from build123d import *

# Parameters (mm, degrees)
SKETCH1_W            = 70
SKETCH1_H            = 40
BOSS_EXTRUDE1_DEPTH  = 5
SKETCH2_W            = 90
SKETCH2_H            = 40
BOSS_EXTRUDE2_DEPTH  = 3
M3_CLEARANCE_HOLE1_D = 3.6
M3_CLEARANCE_HOLE2_D = 3.4
SKETCH9_R            = 14
CUT_EXTRUDE1_DEPTH   = 50.889878733
SKETCH10_W           = 40
SKETCH10_H           = 5
CUT_EXTRUDE2_DEPTH   = 0.5


with BuildPart() as part:
    # Sketch1 → Boss-Extrude1 (new body)
    with BuildSketch(Plane(origin=(0, 0, 0), x_dir=(1, 0, 0), z_dir=(0, 1, 0))):
        Rectangle(SKETCH1_W, SKETCH1_H)
    extrude(amount=BOSS_EXTRUDE1_DEPTH)

    # Sketch2 → Boss-Extrude2 (add)
    with BuildSketch(Plane.XZ):
        Rectangle(SKETCH2_W, SKETCH2_H)
    extrude(amount=BOSS_EXTRUDE2_DEPTH)

    # M3 Clearance Hole1 (through all)
    with Locations(Plane(origin=(0, 0, 0), x_dir=(1, 0, 0), z_dir=(0, 1, 0))):
        with Locations((-40, 15), (-40, -15), (40, 15), (40, -15)):
            Hole(M3_CLEARANCE_HOLE1_D / 2)

    # M3 Clearance Hole2 (through all)
    with Locations(Plane(origin=(0, 5, 0), x_dir=(1, 0, 0), z_dir=(0, 1, 0))):
        with Locations((0, 0), (15.25, 15.25), (-15.25, -15.25), (-15.25, 15.25), (15.25, -15.25)):
            Hole(M3_CLEARANCE_HOLE2_D / 2)

    # Sketch9 → Cut-Extrude1 (cut, through all)
    with BuildSketch(Plane(origin=(0, 5, 0), x_dir=(1, 0, 0), z_dir=(0, 1, 0))):
        with Locations(Location((0, 0, 0), (0, 0, 270))):
            Circle(SKETCH9_R)
    extrude(amount=-CUT_EXTRUDE1_DEPTH, mode=Mode.SUBTRACT)

    # Sketch10 → Cut-Extrude2 (cut)
    with BuildSketch(Plane.ZY.offset(35)):
        with Locations((0, 2.5)):
            Rectangle(SKETCH10_W, SKETCH10_H)
    cut_extrude2 = extrude(amount=-CUT_EXTRUDE2_DEPTH, mode=Mode.SUBTRACT)

    # Mirror1: Cut-Extrude2 across plane
    add(cut_extrude2.mirror(Plane(origin=(0, 0, 0), x_dir=(0, 0, 1), z_dir=(1, 0, 0))), mode=Mode.SUBTRACT)


solid = part.part
Geometry check sheet. Reference: the model listing, model coordinates, mm. A direction names the side the tool comes from. Round coordinates to 2 decimals unless told otherwise and drop trailing zeros. Loops run counter-clockwise (first coordinate to the right, second up) from the corner with the lowest first, then second, coordinate; pieces in that order, holes last.
Item 1: Cross-section at D-D on x = -8.5. Record the boundary of the cut face in (y, z), then the cut area to 3 significant figures.
Item 2: Cross-section at B-B on y = 1.75. Record the boundary of the cut face in (x, z), then the cut area to 3 significant figures.
Item 3: Thickness scan on line 1 (Z direction, x = 15, y = 2.25); line 2 (Z direction, x = -40, y = -1.5); line 3 (X direction, y = -1.35, z = 15). Record the ranges inside material, lowest first.
Item 4: Access from +Z, -Z, +X, -X, +Y, -Y to the whole of each face (thin tool, end or side, straight path). Record for faces 5 (the flat face through (-40, 0, 0)), 6 (the flat face through (40, 0, 0)), 7 (the flat face through (45, -1, 0)).
Item 5: Cross-section at A-A on x = -40. Record the boundary of the cut face in (y, z).
Item 6: Cross-section at C-C on z = 0. Record the boundary of the cut face in (x, y).
Item 7: Mould release check, pull along Z, two halves, no side actions. Record for faces 1 (the flat face through (-1, 1, 20)), 2 (the flat face through (34.5, 3, 0)), 3 (the cylindrical face through (-40.968, -1.521, -16.518)), 4 (the cylindrical face through (39.032, -1.521, 13.482)): pulls with the +Z half, pulls with the -Z half, needs draft (parallel to the pull), parting line crosses it, or undercut.
Item 8: Gauge pin test, flat ends, axial feed: pin 1 (8.5 mm diameter, centred on x = -39, z = -0.5, fed in from +Y); pin 2 (1 mm diameter, centred on y = 3.5, z = 13, fed in from +X); pin 3 (1.5 mm diameter, centred on y = 1.5, z = 1.5, fed in from -X). Record the tip position at first contact, or that the pin passes through.
Answer sheet:
1. outline: (-3, -20) - (5, -20) - (5, -11.12) - (-3, -11.12) - close; (-3, 11.12) - (5, 11.12) - (5, 20) - (-3, 20) - close
1. area: 142 mm2
2. outline: (-34.5, -20) - (34.5, -20) - (34.5, 20) - (-34.5, 20) - close; hole circle Ø3.4 at (-15.25, -15.25); hole circle Ø3.4 at (-15.25, 15.25); hole circle Ø28 at (0, 0); hole circle Ø3.4 at (15.25, -15.25); hole circle Ø3.4 at (15.25, 15.25)
2. area: 2,110 mm2
3. line 1: z = -20 to -16.93, -13.57 to 13.57, 16.93 to 20
3. line 2: z = -20 to -16.8, -13.2 to 13.2, 16.8 to 20
3. line 3: x = -45 to -41.8, -38.2 to -16.93, -13.57 to 13.57, 16.93 to 38.2, 41.8 to 45
4. face 5: +Z, -Z, -X, +Y
4. face 6: +Z, -Z, +X, +Y
4. face 7: +Z, -Z, +X, +Y, -Y
5. outline: (-3, -20) - (0, -20) - (0, -16.8) - (-3, -16.8) - close; (-3, -13.2) - (0, -13.2) - (0, 13.2) - (-3, 13.2) - close; (-3, 16.8) - (0, 16.8) - (0, 20) - (-3, 20) - close
6. outline: (-45, -3) - (-14, -3) - (-14, 5) - (-34.5, 5) - (-34.5, 0) - (-45, 0) - close; (14, -3) - (45, -3) - (45, 0) - (34.5, 0) - (34.5, 5) - (14, 5) - close
7. face 1: pulls with the +Z half
7. face 2: needs draft
7. face 3: undercut
7. face 4: undercut
8. pin 1: stops at y = 0
8. pin 2: stops at x = 34.5
8. pin 3: stops at x = -34.5
